Autodesk Inventor part; units mm, degrees
ref_plane "YZ Plane" through (0, 0, 0) normal (1, 0, 0) x (0, 1, 0)
ref_plane "XZ Plane" through (0, 0, 0) normal (0, 1, 0) x (-1, 0, 0)
ref_plane "XY Plane" through (0, 0, 0) normal (0, 0, 1) x (1, 0, 0)
sketch "Sketch1" plane through (0, 0, 0) normal (0, 0, 1) x (1, 0, 0)
  circle A0 centre (-10.2325, -6.35) radius 2
  circle A1 centre (-10.2325, 6.35) radius 2
  circle A2 centre (10.0875, 6.35) radius 2
  circle A3 centre (10.0875, -6.35) radius 2
  line L0 (-15.3125, 10.2775) -> (10.2325, 10.2775)
  line L1 (10.2325, 10.2775) -> (15.3125, 10.2775)
  line L2 (15.3125, 10.2775) -> (15.3125, -10.2775)
  line L3 (-15.3125, 10.2775) -> (-15.3125, -10.2775)
  line L4 (-15.3125, -10.2775) -> (15.3125, -10.2775)
  line L5 (0, -10.2775) -> (0, 10.2775)
  line L6 (-15.3125, 0) -> (0, 0)
  point P0 (0, 0)
  dimension "d1" = 5.08
extrude "Extrusion1" add sketch "Sketch1" along normal blind 3.81 contours A0 | A1 | A2 | A3 | L0 L5 L6 L3 | L0 L1 L2 L4 L5 | L6 L5 L4 L3
sketch "Sketch2" plane through (0, 0, 3.81) normal (0, 0, 1) x (1, 0, 0)
  line L0 (-15.3125, -10.2775) -> (15.3125, -10.2775)
  line L1 (15.3125, -10.2775) -> (15.3125, 10.2775)
  line L2 (15.3125, 10.2775) -> (-15.3125, 10.2775)
  line L3 (-15.3125, 10.2775) -> (-15.3125, -10.2775)
  point P0 (0, 0)
extrude "Extrusion2" add sketch "Sketch2" along normal blind 1.5875
sketch "Sketch3" plane through (0, 0, 5.3975) normal (0, 0, 1) x (1, 0, 0)
  circle A0 centre (-10.2325, -6.35) radius 2
  circle A1 centre (10.0875, -6.35) radius 2
  circle A2 centre (10.0875, 6.35) radius 2
  circle A3 centre (-10.2325, 6.35) radius 2
  line L0 (-15.3125, -10.2775) -> (15.3125, -10.2775)
  line L1 (10.0875, -10.2775) -> (10.0875, 10.2775)
  line L2 (15.3125, 10.2775) -> (-15.3125, 10.2775)
  line L3 (-10.2325, -10.2775) -> (-10.2325, 10.2775)
  line L4 (-10.2325, 10.2775) -> (10.0875, 10.2775)
  line L5 (10.0875, -10.2775) -> (-10.2325, -10.2775)
  line L6 (15.3125, -10.2775) -> (15.3125, 10.2775)
  point P0 (0, 0)
extrude "Extrusion3" add sketch "Sketch3" along normal blind 8.9916 contours A0 L3 | A0 L3 A3 L2 L1 A2 A1 L0 | L3 A3 | A1 L1 | L1 A2 picked at (-9.5825, -6.2017) picked at (-9.5825, 6.4983) picked at (9.4642, -6.5864) picked at (9.4642, 6.1136)
sketch "Sketch4" plane through (-10.2325, -10.2775, 5.3975) normal (-1, 0, 0) x (0, 0, 1)
  line L0 (8.9916, 20.555) -> (8.9916, 0)
  line L1 (8.9916, 10.2775) -> (0, 10.2775)
  line L2 (0, 0) -> (0, 20.555)
  line L3 (4.4958, 10.2775) -> (4.4958, 5.7817)
  line L4 (4.4958, 10.2775) -> (4.4958, 14.7733)
  circle A0 centre (4.4958, 5.7817) radius 2
  circle A1 centre (4.4958, 14.7733) radius 2
  point P0 (-5.3975, 10.2775)
  dimension "d8" = 4.4958
  dimension "d9" = 4.4958
  dimension "d10" = 4
  dimension "d11" = 4
extrude "Extrusion4" cut sketch "Sketch4" against normal through all
sketch "Sketch7" plane through (10.0875, -10.2775, 5.3975) normal (1, 0, 0) x (0, 0, -1)
  line L0 (0, 20.555) -> (0, 0)
  line L1 (0, 20.555) -> (-8.9916, 20.555)
  line L2 (-8.9916, 0) -> (-8.9916, 20.555)
  line L3 (0, 0) -> (-8.9916, 0)
  point P0 (5.3975, 10.2775)
extrude "Extrusion7" cut sketch "Sketch7" against normal blind 6.289
fillet "Fillet5" radius 3.175 8 edges at (-15.3125, 10.2775, 2.6987) (-15.3125, -10.2775, 2.6987) (15.3125, 10.2775, 2.6987) (15.3125, -10.2775, 2.6987) (3.7984, 10.2775, 9.8933) (-10.2325, 10.2775, 9.8933) (3.7984, -10.2775, 9.8933) (-10.2325, -10.2775, 9.8933)
sketch "Sketch9" plane through (0, 0, 0) normal (0, 0, -1) x (-1, 0, 0)
  line L0 (-34.8064, -15.875) -> (-34.8064, 15.875)
  line L1 (-27.8064, -15.875) -> (-34.8064, -15.875)
  line L2 (-27.8064, -12.5) -> (-27.8064, -15.875)
  line L3 (-27.8064, 12.5) -> (-27.8064, -12.5)
  line L4 (-27.8064, 15.875) -> (-27.8064, 12.5)
  line L5 (-34.8064, 15.875) -> (-27.8064, 15.875)
  line L6 (-27.8064, 12.5) -> (-27.8064, -12.5)
  line L7 (-27.8064, -12.5) -> (27.1936, -12.5)
  line L8 (27.1936, 12.5) -> (27.1936, -12.5)
  line L9 (27.1936, 12.5) -> (-27.8064, 12.5)
  line L10 (-34.8064, 0) -> (-27.8064, 0)
  line L11 (-31.3064, 0) -> (-31.3064, -6.985)
  line L12 (-31.3064, 0) -> (-31.3064, 6.985)
  circle A0 centre (-31.3064, -6.985) radius 1.5
  circle A1 centre (-31.3064, 6.985) radius 1.5
  circle A2 centre (23.6936, -6.985) radius 1.5
  circle A3 centre (23.6936, 6.985) radius 1.5
  line L13 (-34.8064, 0) -> (27.1936, 0)
  line L14 (0, 0) -> (0, 12.5)
  point P0 (0, 0)
  point P1 (-34.8064, 0)
  point P2 (-34.8064, 0)
  dimension "d26" = 6.985
  dimension "d27" = 6.985
  dimension "d28" = 3
  dimension "d29" = 3
extrude "Extrusion9" cut sketch "Sketch9" against normal up to surface (5.3975 mm away) contours L3 L13 L8 L7 | L3 L9 L14 L13 | L14 L9 L8 L13
sketch "Sketch10" plane through (0.6234, 10.2775, 5.3975) normal (0, 0, -1) x (-1, 0, 0)
  line L0 (10.856, -12.7733) -> (10.856, -16.7733)
  line L1 (10.856, -3.7817) -> (10.856, -7.7817)
  arc A0 (0, 0) -> (-3.175, -3.175) centre (0, -3.175) ccw
  arc A1 (0, 0) -> (-3.175, -3.175) centre (0, -3.175) ccw
  arc A2 (0, 0) -> (-3.175, -3.175) centre (0, -3.175) ccw
  arc A3 (0, 0) -> (-3.175, -3.175) centre (0, -3.175) ccw
  arc A4 (10.856, -3.175) -> (7.681, 0) centre (7.681, -3.175) ccw
  arc A5 (10.856, -3.175) -> (7.681, 0) centre (7.681, -3.175) ccw
  arc A6 (10.856, -3.175) -> (7.681, 0) centre (7.681, -3.175) ccw
  line L2 (-3.175, -3.7817) -> (-3.175, -7.7817)
  line L3 (-3.175, -3.7817) -> (-3.175, -7.7817)
  line L4 (10.856, -3.7817) -> (10.856, -7.7817)
  line L5 (-3.175, -12.7733) -> (-3.175, -16.7733)
  line L6 (-3.175, -17.38) -> (-3.175, -3.175)
  line L7 (-3.175, -3.175) -> (-3.175, -17.38)
  line L8 (-3.175, -17.38) -> (-3.175, -3.175)
  line L9 (-3.175, -3.7817) -> (-3.175, -7.7817)
  line L10 (-3.175, -12.7733) -> (-3.175, -16.7733)
  line L11 (-3.175, -3.175) -> (-3.175, -17.38)
  line L12 (10.856, -3.175) -> (10.856, -17.38)
  line L13 (10.856, -17.38) -> (10.856, -3.175)
  line L14 (10.856, -3.175) -> (10.856, -17.38)
  line L15 (10.856, -17.38) -> (10.856, -3.175)
  line L16 (10.856, -3.7817) -> (10.856, -7.7817)
  line L17 (10.856, -12.7733) -> (10.856, -16.7733)
  line L18 (-3.175, -12.7733) -> (-3.175, -16.7733)
  line L19 (10.856, -12.7733) -> (10.856, -16.7733)
  line L20 (7.681, -20.555) -> (0, -20.555)
  line L21 (7.681, -20.555) -> (0, -20.555)
  line L22 (7.681, -20.555) -> (0, -20.555)
  line L23 (7.681, -20.555) -> (0, -20.555)
  arc A7 (-3.175, -17.38) -> (0, -20.555) centre (0, -17.38) ccw
  arc A8 (-3.175, -17.38) -> (0, -20.555) centre (0, -17.38) ccw
  arc A9 (-3.175, -17.38) -> (0, -20.555) centre (0, -17.38) ccw
  arc A10 (7.681, -20.555) -> (10.856, -17.38) centre (7.681, -17.38) ccw
  arc A11 (7.681, -20.555) -> (10.856, -17.38) centre (7.681, -17.38) ccw
  line L24 (0, 0) -> (7.681, 0)
  arc A12 (0, 0) -> (-3.175, -3.175) centre (0, -3.175) ccw
  line L25 (-3.175, -3.175) -> (-3.175, -17.38)
  arc A13 (-3.175, -17.38) -> (0, -20.555) centre (0, -17.38) ccw
  line L26 (7.681, -20.555) -> (0, -20.555)
  arc A14 (7.681, -20.555) -> (10.856, -17.38) centre (7.681, -17.38) ccw
  line L27 (10.856, -17.38) -> (10.856, -3.175)
  arc A15 (10.856, -3.175) -> (7.681, 0) centre (7.681, -3.175) ccw
  arc A16 (-3.175, -17.38) -> (0, -20.555) centre (0, -17.38) ccw
  arc A17 (7.681, -20.555) -> (10.856, -17.38) centre (7.681, -17.38) ccw
  arc A18 (7.681, -20.555) -> (10.856, -17.38) centre (7.681, -17.38) ccw
  line L28 (7.681, -20.555) -> (0, -20.555)
  arc A19 (-3.175, -17.38) -> (0, -20.555) centre (0, -17.38) ccw
  line L29 (-3.175, -17.38) -> (-3.175, -3.175)
  arc A20 (0, 0) -> (-3.175, -3.175) centre (0, -3.175) ccw
  line L30 (0, 0) -> (7.681, 0)
  arc A21 (10.856, -3.175) -> (7.681, 0) centre (7.681, -3.175) ccw
  line L31 (10.856, -3.175) -> (10.856, -17.38)
  line L32 (0, 0) -> (7.681, 0)
  line L33 (0, 0) -> (7.681, 0)
  line L34 (0, 0) -> (7.681, 0)
  line L35 (0, 0) -> (7.681, 0)
  arc A22 (10.856, -3.175) -> (7.681, 0) centre (7.681, -3.175) ccw
  arc A23 (7.681, -20.555) -> (10.856, -17.38) centre (7.681, -17.38) ccw
  line L36 (0.6234, -10.2775) -> (0.6234, 2.2225)
  line L37 (0.6234, -10.2775) -> (-1.4597, -6.785)
  line L38 (8.1734, -10.2775) -> (-23.133, -10.2775)
  line L39 (-21.538, 5.5975) -> (-21.538, -26.1525)
  line L40 (-21.538, -26.1525) -> (-28.538, -26.1525)
  line L41 (-28.538, -26.1525) -> (-28.538, 5.5975)
  line L42 (-21.538, 5.5975) -> (-28.538, 5.5975)
  circle A24 centre (-25.038, -3.2925) radius 1.5
  circle A25 centre (-25.038, -17.2625) radius 1.5
  line L43 (-25.038, -10.2775) -> (-25.038, -17.2625)
  line L44 (-23.133, -10.2775) -> (-25.038, -10.2775)
  line L45 (-27.133, -22.7775) -> (-29.038, -22.7775)
  line L46 (-27.133, 2.2225) -> (-29.038, 2.2225)
  line L47 (0.6234, -10.2775) -> (2.7066, -13.77)
  line L48 (-21.538, -22.7775) -> (35.367, -22.7775)
  line L49 (35.367, -22.7775) -> (35.367, 2.2225)
  line L50 (35.367, 2.2225) -> (-21.538, 2.2225)
  circle A26 centre (31.867, -17.2625) radius 1.5
  circle A27 centre (31.867, -3.2925) radius 1.5
  line L51 (0.6234, -10.2775) -> (8.1734, -10.2775)
  point P0 (0.6234, -10.2775)
  point P1 (0.6234, -10.2775)
  point P2 (0, 0)
  dimension "d47" = 1.905
  dimension "d48" = 7.55
extrude "Extrusion10" add sketch "Sketch10" along normal blind 9
fillet "Fillet17" radius 3.81 4 edges at (29.1614, -15.875, 0.8975) (-34.7436, -12.5, 0.8975) (-34.7436, 12.5, 0.8975) (29.1614, 15.875, 0.8975)
fillet "Fillet18" radius 3.175 2 edges at (22.1614, -15.875, 0.8975) (22.1614, 15.875, 0.8975)
fillet "Fillet19" radius 3.175 2 edges at (22.1614, -12.5, 0.8975) (22.1614, 12.5, 0.8975)
sketch "Sketch11" plane through (0, 0, 14.3891) normal (0, 0, 1) x (1, 0, 0)
  arc A0 (-10.2325, -7.1025) -> (-7.0575, -10.2775) centre (-7.0575, -7.1025) ccw
  line L0 (-7.0575, -10.2775) -> (0.6234, -10.2775)
  arc A1 (0.6234, -10.2775) -> (3.7984, -7.1025) centre (0.6234, -7.1025) ccw
  line L1 (3.7984, -7.1025) -> (3.7984, 7.1025)
  arc A2 (3.7984, 7.1025) -> (0.6234, 10.2775) centre (0.6234, 7.1025) ccw
  line L2 (0.6234, 10.2775) -> (-7.0575, 10.2775)
  arc A3 (-7.0575, 10.2775) -> (-10.2325, 7.1025) centre (-7.0575, 7.1025) ccw
  line L3 (-10.2325, 7.1025) -> (-10.2325, -7.1025)
  arc A4 (-82.2091, -59.7824) -> (-79.0341, -62.9574) centre (-79.0341, -59.7824) ccw
  line L4 (-79.0341, -62.9574) -> (-71.3531, -62.9574)
  arc A5 (-71.3531, -62.9574) -> (-68.1781, -59.7824) centre (-71.3531, -59.7824) ccw
  line L5 (-68.1781, -59.7824) -> (-68.1781, -45.5774)
  arc A6 (-68.1781, -45.5774) -> (-71.3531, -42.4024) centre (-71.3531, -45.5774) ccw
  line L6 (-71.3531, -42.4024) -> (-79.0341, -42.4024)
  arc A7 (-79.0341, -42.4024) -> (-82.2091, -45.5774) centre (-79.0341, -45.5774) ccw
  line L7 (-82.2091, -45.5774) -> (-82.2091, -59.7824)
  point P0 (-71.9766, -52.6799)
extrude "Extrusion11" cut sketch "Sketch11" against normal up to surface (8.9916 mm away) contours L3 A3 L2 A2 L1 A1 L0 A0
fillet "Fillet23" radius 3.175 14 edges at (21.3632, 12.9544, -3.6025) (23.6997, 15.4206, -3.6025) (25.3439, 15.875, -3.6025) (28.0455, 14.7591, -3.6025) (29.1614, 0, -3.6025) (28.0455, -14.7591, -3.6025) (25.3439, -15.875, -3.6025) (23.6997, -15.4206, -3.6025) (21.3632, -12.9544, -3.6025) (-5.6036, -12.5, -3.6025) (-33.6277, -11.3841, -3.6025) (-34.7436, 0, -3.6025) (-33.6277, 11.3841, -3.6025) (-5.6036, 12.5, -3.6025)
sketch "Sketch14" plane through (0.6234, 10.2775, -3.6025) normal (0, 0, -1) x (-1, 0, 0)
  circle A0 centre (3.4145, -17.0275) radius 1.5
  circle A1 centre (3.4145, -10.2775) radius 1.5
  circle A2 centre (3.4145, -3.5275) radius 1.5
  line L0 (-28.538, 1.7875) -> (-28.538, -22.3425)
  line L1 (-28.538, -10.2775) -> (35.367, -10.2775)
  line L2 (35.367, -18.9675) -> (35.367, -1.5875)
  line L3 (3.4145, -10.2775) -> (3.4145, 9.7711)
  point P0 (0.6234, -10.2775)
extrude "Extrusion14" cut sketch "Sketch14" against normal blind 25.4
properties part number "connecting plate servo flat v5"
CAD build for the part. Positions are in the model's coordinates, mm. A direction names the side the tool comes from. Give positions to 0.01 mm unless a question says otherwise; leave off trailing zeros. Answer in a Markdown table with one row per item. Add a question column.
Item 1: Tool access for faces 1 (the face through (-5, -12.5, 3)), 2 (the face through (-5.25, -11.59, -2.65)), 3 (the face through (-5.249, 11.545, -2.697)): list every direction of +Z, -Z, +X, -X, +Y, -Y with a clear straight run to the whole face (end or side of a thin tool).
Item 2: Mould opens along X. For faces 4 (the face through (-2, 3, -3.602)), 5 (the face through (23.72, -15.433, 2.444)), 6 (the face through (-2.466, 5.286, 0.835)) say: +X half, -X half, draft (parallel to the pull), parting line (faces both ways), or undercut.
Item 3: Probe probe 1 along Y at (x, z) = (-3, 0.5); probe 2 along X at (y, z) = (6.5, -3); probe 3 along X at (y, z) = (0, 3.25). List the from-to ranges inside material, lowest first.
Item 4: Drop flat-ended pins along their axis: P1, Ø1.7, axis at x = -5.5, z = 2, coming from the -Y side; P2, Ø3, axis at x = -23, z = 2.5, coming from the +Y side. Give the stop position or say it passes through.
Item 5: Band-saw the part on A-A on z = 1.75. Give the number of separate pieces and of enclosed holes in the cut face, then the cut area to 3 significant figures.
Reply:
| question | item | result |
|---|---|---|
| 1 | face 1 | +Z, -Z, -X, -Y |
| 1 | face 2 | -Z, -X, -Y |
| 1 | face 3 | -Z, -X, +Y |
| 2 | face 4 | draft |
| 2 | face 5 | -X half |
| 2 | face 6 | undercut |
| 3 | probe 1 | y = -12.5 to -8.24, -5.26 to -1.49, 1.49 to 5.26, 8.24 to 12.5 |
| 3 | probe 2 | x = -33.43 to -32.66, -29.82 to -4.27, -1.31 to 24.24, 27.08 to 27.85 |
| 3 | probe 3 | x = -34.74 to -4.29, -1.29 to 29.16 |
| 4 | P1 | stops at y = -12.5 |
| 4 | P2 | stops at y = 12.5 |
| 5 | separate pieces | 1 |
| 5 | enclosed holes | 7 |
| 5 | area | 1,580 mm^2 |
